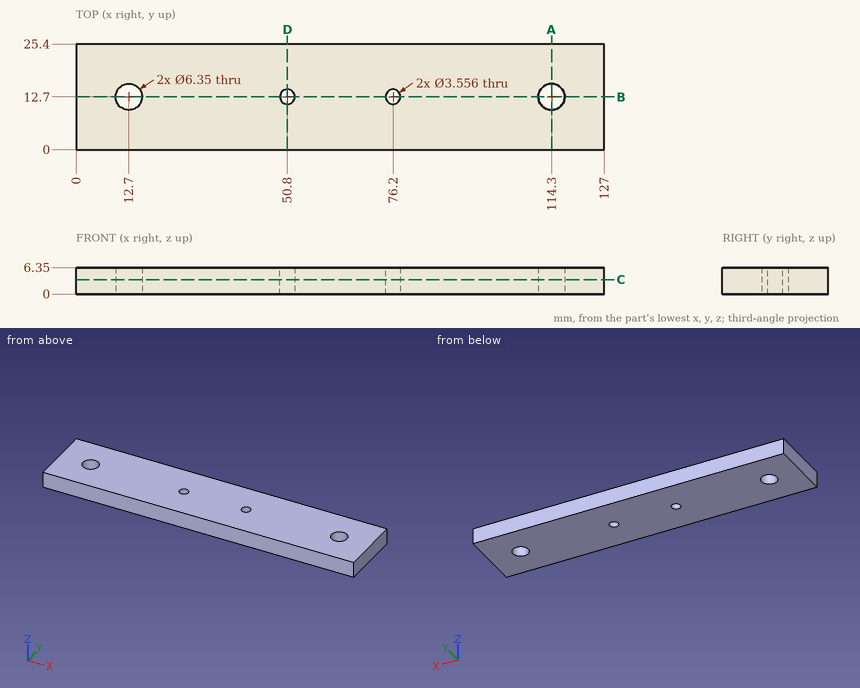
Here's the drawing with two shaded views (mm, measured from the low corner). I have some questions. Round coordinates to 2 decimals unless told otherwise and drop trailing zeros. Loops run counter-clockwise (first coordinate to the right, second up) from the corner with the lowest first, then second, coordinate; pieces in that order, holes last. Notation, with made-up numbers: (-25.5, 12) - (-5.5, 12) arc R23 ccw to (-5.5, 48) - close; hole circle Ø3 at (20.25, 42). An arc over 180 degrees is marked (long way). Write item = value, one per line.
1) Imagine slicing it at A-A (x = 114.3). Please give me the cut outline in (y, z) (3 decimals), and give its area (3 significant figures).
Computed:
outline = (0, 0) - (9.525, 0) - (9.525, 6.35) - (0, 6.35) - close; (15.875, 0) - (25.4, 0) - (25.4, 6.35) - (15.875, 6.35) - close
area = 121 mm2
2) Imagine slicing it at B-B (y = 12.7). Please give me the cut outline in (x, z) (3 decimals), and give its area (3 significant figures).
Computed:
outline = (0, 0) - (9.525, 0) - (9.525, 6.35) - (0, 6.35) - close; (15.875, 0) - (49.022, 0) - (49.022, 6.35) - (15.875, 6.35) - close; (52.578, 0) - (74.422, 0) - (74.422, 6.35) - (52.578, 6.35) - close; (77.978, 0) - (111.125, 0) - (111.125, 6.35) - (77.978, 6.35) - close; (117.475, 0) - (127, 0) - (127, 6.35) - (117.475, 6.35) - close
area = 681 mm2
3) Imagine slicing it at D-D (x = 50.8). Please give me the cut outline in (y, z), and give its area (3 significant figures).
Computed:
outline = (0, 0) - (10.92, 0) - (10.92, 6.35) - (0, 6.35) - close; (14.48, 0) - (25.4, 0) - (25.4, 6.35) - (14.48, 6.35) - close
area = 139 mm2
4) Imagine slicing it at C-C (z = 3.5). Please give me the cut outline in (x, y) (3 decimals), and give its area (3 significant figures).
Computed:
outline = (0, 0) - (127, 0) - (127, 25.4) - (0, 25.4) - close; hole circle Ø6.35 at (12.7, 12.7); hole circle Ø3.556 at (50.8, 12.7); hole circle Ø3.556 at (76.2, 12.7); hole circle Ø6.35 at (114.3, 12.7)
area = 3,140 mm2
5) I'm going to push a flat-ended pin straight in: P1, Ø1.5, axis at x = 15, y = 15.5, coming from the -Z side. Where does the tip first touch, or does it pass through?
Computed:
P1 = 0
6) I need wall thicknesses on line 1 along Y through (x, z) = (76.2, 2.5); line 2 along Y through (x, z) = (12.7, 4.75) (3 decimals). Which ranges of each line are inside material? Lowest first, please. Write a range as from..to.
Computed:
line_1 = 0..10.92, 14.48..25.4
line_2 = 0..9.525, 15.875..25.4
